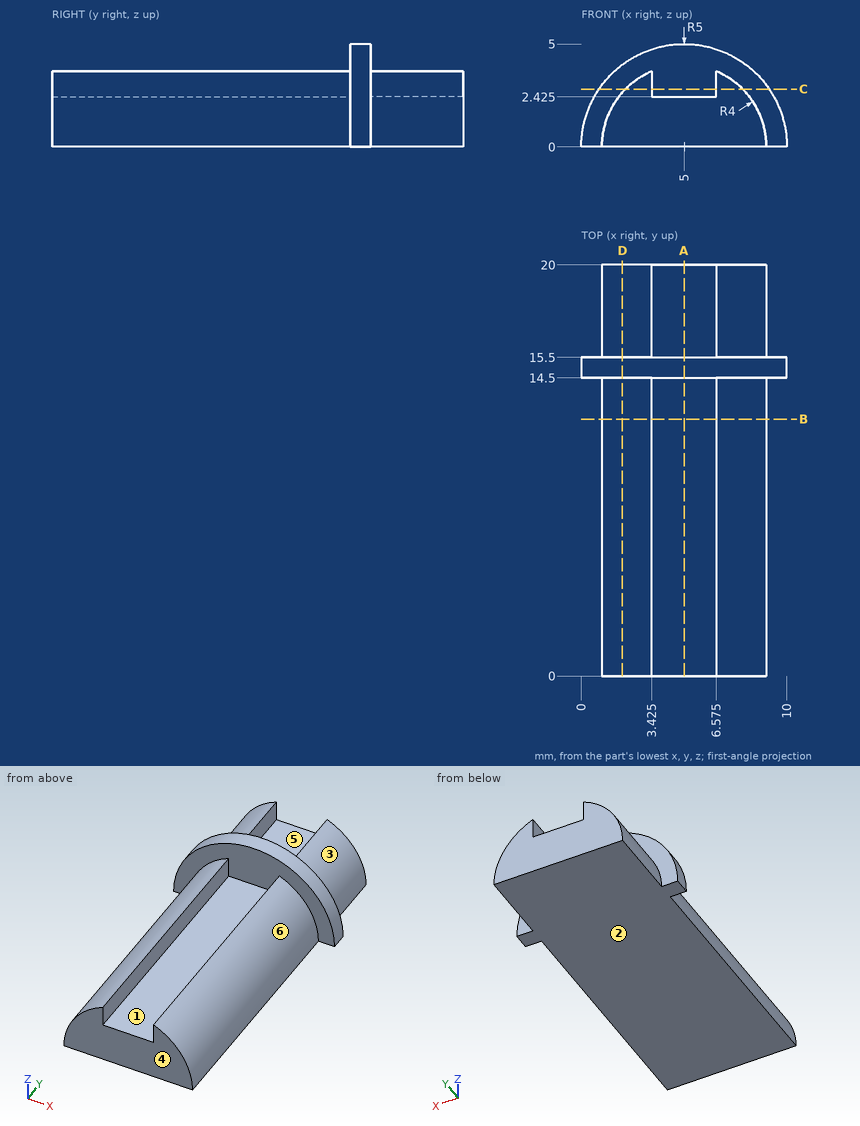
Geometry: see drawing. Coordinates: mm, zero at the bounding-box minimum. A direction names the side the tool comes from. Coordinates: 2 decimals unless noted, no trailing zeros. Loops run counter-clockwise (first coordinate to the right, second up) from the corner with the lowest first, then second, coordinate; pieces in that order, holes last. Notation, with made-up numbers: (80, -5) - (110, -5) arc R37 ccw to (110, 31) - close; hole circle Ø9 at (18.5, 56.25). An arc over 180 degrees is marked (long way). Return JSON: item names as keys, results as strings.
Q1. Section C-C, the plane z = 2.8. Return loops of the section in (x, y) (3 decimals), plus the area to 3 significant figures.
Results:
{"outline": "(0.858, 14.5) - (2.143, 14.5) - (2.143, 0) - (3.425, 0) - (3.425, 14.5) - (6.575, 14.5) - (6.575, 0) - (7.857, 0) - (7.857, 14.5) - (9.142, 14.5) - (9.142, 15.5) - (7.857, 15.5) - (7.857, 20) - (6.575, 20) - (6.575, 15.5) - (3.425, 15.5) - (3.425, 20) - (2.143, 20) - (2.143, 15.5) - (0.858, 15.5) - close", "area": "57.0 mm2"}
Q2. Section A-A, the plane x = 5. Return loops of the section in (y, z) (3 decimals).
Results:
{"outline": "(0, 0) - (20, 0) - (20, 2.425) - (15.5, 2.425) - (15.5, 5) - (14.5, 5) - (14.5, 2.425) - (0, 2.425) - close"}
Q3. Mould query, pull axis X, two halves, no side actions, for the marked faces 1, 2 and 3. Classes: released by +X, released by -X, zero draft, split by the parting line, or undercut.
Results:
{"face 1": "undercut", "face 2": "zero draft", "face 3": "released by +X"}
Q4. Access query for the marked faces 4, 5 and 6. Directions: +Z, -Z, +X, -X, +Y, -Y. A direction counts if a zero-diameter tool reaches every point of the face in a straight line with its end or side. Return the directions, or none.
Results:
{"face 4": "+Z, -Z, +X, -X, -Y", "face 5": "+Z, +Y", "face 6": "+Z, +X, -Y"}
Q5. Contact query for flat-ended pins moving along their axis: P1, Ø1, axis at x = 6, y = 2, coming from the +Z side (3 decimals); P2, Ø0.6, axis at y = 10, z = 3.5, coming from the +X side; P3, Ø3.5, axis at x = 5, y = 4, coming from the +Z side. Output: stop coordinate, or through.
Results:
{"P1": "z = 2.425", "P2": "x = 7.4", "P3": "z = 3.68"}
Q6. Section D-D, the plane x = 2. Return loops of the section in (y, z), plus the area to 3 significant figures.
Results:
{"outline": "(0, 0) - (20, 0) - (20, 2.65) - (15.5, 2.65) - (15.5, 4) - (14.5, 4) - (14.5, 2.65) - (0, 2.65) - close", "area": "54.3 mm2"}
Q7. Section B-B, the plane y = 12.5. Return loops of the section in (x, z) (3 decimals), plus the area to 3 significant figures.
Results:
{"outline": "(1, 0) - (9, 0) arc R4 ccw to (6.575, 3.677) - (6.575, 2.425) - (3.425, 2.425) - (3.425, 3.677) arc R4 ccw to start", "area": "20.5 mm2"}
Q8. Material intervals for line 1 along Z through (x, y) = (6, 7.75) (3 decimals); line 2 along Y through (x, z) = (6.25, 2.7); line 3 along X through (y, z) = (8.75, 1.85), sorted ascending.
Results:
{"line 1": "0 to 2.425", "line 2": "14.5 to 15.5", "line 3": "1.45 to 8.55"}
